```python
from build123d import *

# Parameters (mm, degrees)
F0_W          = 50.8
F0_H          = 7.62
F1_DEPTH      = 2.54
F2_R          = 1.905
F3_DEPTH      = 38.1
F5_DEPTH      = 50.801
F5_DEPTH_BACK = 94


# Not quite as in the source:
# - an extrude ends at something that could not be found from the text; its depth is read off the source's solid


with BuildPart() as f1:
    # F0 (on Top) → F1 (new body)
    with BuildSketch(Plane.XY):
        with Locations((25.4, 3.81)):
            Rectangle(F0_W, F0_H)
    extrude(amount=F1_DEPTH)

    # F2 (on face) → F3 (join)
    with BuildSketch(Plane.XY.offset(2.54)):
        with Locations((2.032, 3.81)):
            Circle(F2_R)
        with Locations((48.768, 3.81)):
            Circle(F2_R)
    extrude(amount=F3_DEPTH)

    # F4 (on Right) → F5 (cut, two sides)
    with BuildSketch(Plane.YZ) as f5_sk:
        Polygon((0, 40.64), (0, 38.7614695235), (7.5709112298, 40.7900890735), align=None)
    extrude(amount=F5_DEPTH, mode=Mode.SUBTRACT)
    extrude(f5_sk.sketch, amount=-F5_DEPTH_BACK, mode=Mode.SUBTRACT)


solid = f1.part
```
Read the model definition and answer for the solid it produces. Units are mm, in the model's axes. A direction names the side the tool comes from. Round coordinates to 2 decimals unless told otherwise and drop trailing zeros. Loops run counter-clockwise (first coordinate to the right, second up) from the corner with the lowest first, then second, coordinate; pieces in that order, holes last. Notation, with made-up numbers: (52.25, 12.25) -> (80.25, 12.25) arc R13 cw to (80.25, 22.25) -> close; hole circle Ø6 at (42.5, 0). An arc over 180 degrees is marked (long way). One line per item, written item: value.
1) Flat-ended cylindrical pins translate along their axes: P1, Ø2.5, axis at x = 16.5, y = 2, coming from the +Z side; P2, Ø1, axis at y = 5.5, z = 9.5, coming from the -X side; P3, Ø3, axis at y = 5.5, z = 18, coming from the -X side. Find the tip coordinate at first contact, or state that the pin passes through.
Answer list:
P1: stops at z = 2.54
P2: stops at x = 0.54
P3: stops at x = 0.14
2) The mould has two halves that part along X. Classify faces 1 (the face through (25, 7.62, 1)), 2 (the face through (50.8, 4, 1)), 3 (the face through (47.364, 5.097, 21.203)), 4 (the face through (25, 4, 2.54)): pulls with the +X half, pulls with the -X half, needs draft (parallel to the pull), parting line crosses it, or undercut.
Answer list:
face 1: needs draft
face 2: pulls with the +X half
face 3: undercut
face 4: undercut
3) For faces 5 (the face through (0, 4, 1)), 6 (the face through (1.8, 5.7, 21.2)), determine the directions among +Z, -Z, +X, -X, +Y, -Y from which every point of the face is accessible in a straight line to the end or side of a thin tool.
Answer list:
face 5: +Z, -Z, -X, +Y, -Y
face 6: +Z
4) A cutting plane is placed at B-B (y = 3.81). Determine the outline of the cut face in (x, z), and give its area (3 significant figures).
Answer list:
outline: (0, 0) -> (50.8, 0) -> (50.8, 2.54) -> (50.67, 2.54) -> (50.67, 39.78) -> (46.86, 39.78) -> (46.86, 2.54) -> (3.94, 2.54) -> (3.94, 39.78) -> (0.13, 39.78) -> (0.13, 2.54) -> (0, 2.54) -> close
area: 413 mm²
5) A cutting plane is placed at A-A (z = 27). Determine the outline of the cut face in (x, y) (3 decimals), and give its area (3 significant figures).
Answer list:
outline: circle Ø3.81 at (2.032, 3.81); circle Ø3.81 at (48.768, 3.81)
area: 22.8 mm²
6) A cutting plane is placed at D-D (y = 6.25). Determine the outline of the cut face in (x, z), and give its area (3 significant figures).
Answer list:
outline: (0, 0) -> (50.8, 0) -> (50.8, 2.54) -> (0, 2.54) -> close
area: 129 mm²
7) Consider L1, parallel to Z at x = 26.5, y = 4.75; L2, parallel to X at y = 4.75, z = 16; L3, parallel to X at y = 5.5, z = 4.5. Determine where each line is inside the solid, lowest interval first. Write a range as [from, to].
Answer list:
L1: z = [0, 2.54]
L2: x = [0.38, 3.69], [47.11, 50.42]
L3: x = [1.15, 2.91], [47.89, 49.65]
8) A cutting plane is placed at C-C (x = 17). Determine the outline of the cut face in (y, z), and give its area (3 significant figures).
Answer list:
outline: (0, 0) -> (7.62, 0) -> (7.62, 2.54) -> (0, 2.54) -> close
area: 19.4 mm²
